from build123d import *

# Parameters (mm, degrees)
SKETCH_1_R          = 36
SKETCH_1_R_2        = 31
EXTRUDE_1_DEPTH     = 121
SKETCH_2_R          = 46
SKETCH_2_R_2        = 31
EXTRUDE_2_DEPTH     = 16
EXTRUDE_START       = 2
SKETCH_3_R          = 36
SKETCH_3_R_2        = 28.5
EXTRUDE_3_DEPTH     = 2
EXTRUDE_START_2     = 3
SKETCH_4_R          = 36
SKETCH_4_R_2        = 17
EXTRUDE_4_DEPTH     = 3
SKETCH_5_R          = 1.8
CUT_EXTRUDE_1_DEPTH = 20


with BuildPart() as part:
    # 草图1 → 凸台-拉伸1 (new body)
    with BuildSketch(Plane(origin=(0, 0, 0), x_dir=(0, 0, -1), z_dir=(1, 0, 0))):
        Circle(SKETCH_1_R)
        Circle(SKETCH_1_R_2, mode=Mode.SUBTRACT)
    extrude(amount=EXTRUDE_1_DEPTH)

    # 草图2 → 凸台-拉伸2 (add)
    with BuildSketch(Plane(origin=(121, 0, 0), x_dir=(0, 0, -1), z_dir=(1, 0, 0))):
        Circle(SKETCH_2_R)
        Circle(SKETCH_2_R_2, mode=Mode.SUBTRACT)
    extrude(amount=EXTRUDE_2_DEPTH)

    # 草图3 → 凸台-拉伸3 (add)
    with BuildSketch(Plane.ZY.offset(EXTRUDE_START)):
        Circle(SKETCH_3_R)
        Circle(SKETCH_3_R_2, mode=Mode.SUBTRACT)
    extrude(amount=-EXTRUDE_3_DEPTH)

    # 草图4 → 凸台-拉伸4 (add)
    with BuildSketch(Plane.ZY.offset(2).offset(EXTRUDE_START_2)):
        Circle(SKETCH_4_R)
        Circle(SKETCH_4_R_2, mode=Mode.SUBTRACT)
    extrude(amount=-EXTRUDE_4_DEPTH)

    # 草图5 → 切除-拉伸1 (cut)
    with BuildSketch(Plane(origin=(137, 0, 0), x_dir=(0, 0, -1), z_dir=(1, 0, 0))):
        with Locations((0, 40)):
            Circle(SKETCH_5_R)
        with Locations((40, 0)):
            Circle(SKETCH_5_R)
        with Locations((0, -40)):
            Circle(SKETCH_5_R)
        with Locations((-40, 0)):
            Circle(SKETCH_5_R)
    extrude(amount=-CUT_EXTRUDE_1_DEPTH, mode=Mode.SUBTRACT)


solid = part.part
Part model, mm, in its own coordinate system. A direction names the side the tool comes from. Coordinates: 2 decimals unless noted, no trailing zeros. Order: outer loops, then holes, each group sorted by start corner. A loop starts at its lowest first (then second) coordinate and runs counter-clockwise, first axis right, second up. Notation, with made-up numbers: M 6.25,-18 L 53.25,-18 A30 cw 53.25,18 Z; hole C -26.5,16.5 d5. An arc over 180 degrees is marked long. Use a Markdown table: item, result.
(1) Tool access for faces 5 (the flat face through (-5, -15.5, 7.5)), 6 (the flat face through (121, 27.5, -23.6)), 7 (the cylindrical face through (67.541, 30.736, 4.036)): list every direction of +Z, -Z, +X, -X, +Y, -Y with a clear straight run to the whole face (end or side of a thin tool).
A:
| item | result |
|---|---|
| face 5 | +Z, -Z, -X, +Y, -Y |
| face 6 | -X |
| face 7 | +X |
(2) Probe L1, parallel to Y at x = 128.75, z = 0; L2, parallel to Y at x = -1.3, z = 0; L3, parallel to Y at x = -4.2, z = 0. List the from-to ranges inside material, lowest first.
A:
| item | result |
|---|---|
| L1 | y = -46 to -41.8, -38.2 to -31, 31 to 38.2, 41.8 to 46 |
| L2 | y = -36 to -28.5, 28.5 to 36 |
| L3 | y = -36 to -17, 17 to 36 |
(3) Cut at A-A on y = 0. Write the cut outline in (x, z), then the cut area to 3 significant figures.
A:
| item | result |
|---|---|
| outline | M -5,-36 L 121,-36 L 121,-38.2 L 137,-38.2 L 137,-31 L 0,-31 L 0,-28.5 L -2,-28.5 L -2,-17 L -5,-17 Z; M -5,17 L -2,17 L -2,28.5 L 0,28.5 L 0,31 L 137,31 L 137,38.2 L 121,38.2 L 121,36 L -5,36 Z; M 121,-46 L 137,-46 L 137,-41.8 L 121,-41.8 Z; M 121,41.8 L 137,41.8 L 137,46 L 121,46 Z |
| area | 1,720 mm^2 |
(4) Flat gauge pins, fed straight in: pin 1 (3 mm diameter, centred on y = -40, z = 0, fed in from -X); pin 2 (4 mm diameter, centred on y = 0, z = -40, fed in from -X); pin 3 (4 mm diameter, centred on x = 76, y = -16.5, fed in from +Z); pin 4 (10 mm diameter, centred on x = 30.5, z = -0.5, fed in from -Y). Where does each tip first touch, or does it go through?
A:
| item | result |
|---|---|
| pin 1 | passes through |
| pin 2 | stops at x = 121 |
| pin 3 | stops at z = 32.95 |
| pin 4 | stops at y = -36 |
(5) Cut at D-D on y = -15. Write the cut outline in (x, z).
A:
| item | result |
|---|---|
| outline | M -5,-32.73 L 121,-32.73 L 121,-43.49 L 137,-43.49 L 137,-27.13 L 0,-27.13 L 0,-24.23 L -2,-24.23 L -2,-8 L -5,-8 Z; M -5,8 L -2,8 L -2,24.23 L 0,24.23 L 0,27.13 L 137,27.13 L 137,43.49 L 121,43.49 L 121,32.73 L -5,32.73 Z |
(6) Pull direction Z, two halves, no side cores. Call faces 1 (the cylindrical face through (128.89, 45.61, 5.99)), 2 (the flat face through (0, -14, 25)), 3 (the cylindrical face through (-3.521, 14.334, 9.139)), 4 (the flat face through (137, -10, -30)): released by +Z, released by -Z, zero draft, split by the parting line, or undercut.
A:
| item | result |
|---|---|
| face 1 | split by the parting line |
| face 2 | undercut |
| face 3 | undercut |
| face 4 | zero draft |
(7) Cut at C-C on z = 40. Write the cut outline in (x, y).
A:
| item | result |
|---|---|
| outline | M 121,-22.72 L 137,-22.72 L 137,-1.8 L 121,-1.8 Z; M 121,1.8 L 137,1.8 L 137,22.72 L 121,22.72 Z |
